```python
from build123d import *

# Parameters (mm, degrees)
F0_W     = 9
F0_H     = 15
F0_W_2   = 3.2
F1_DEPTH = 9
F3_SIZE  = 2


# Not quite as in the source:
# - a feature names something its author has since deleted; it is built from what else it names


with BuildPart() as f1:
    # F0 (on Top) → F1 (new body, symmetric)
    with BuildSketch(Plane.XY):
        with Locations((-4.5, -7.5)):
            Rectangle(F0_W, F0_H)
        with Locations((1.6, -7.5)):
            Rectangle(F0_W_2, F0_H)
        with BuildLine():
            Line((41, 0), (3.2, 0))
            Line((3.2, 0), (3.2, -15))
            Line((3.2, -15), (41, -15))
            ThreePointArc((41, -15), (62.2132034356, -6.2132034356), (71, 15))
            Line((71, 15), (71, 85))
            ThreePointArc((71, 85), (62.2132034356, 106.2132034356), (41, 115))
            Line((41, 115), (-9, 115))
            Line((-9, 115), (-9, 100))
            Line((-9, 100), (41, 100))
            ThreePointArc((41, 100), (51.6066017178, 95.6066017178), (56, 85))
            Line((56, 85), (56, 15))
            ThreePointArc((56, 15), (51.6066017178, 4.3933982822), (41, 0))
        make_face()
    extrude(amount=F1_DEPTH, both=True)

    # F0 (on Top) → F2 (revolve, cut)
    with BuildSketch(Plane.XY):
        with Locations((1.6, -7.5)):
            Rectangle(F0_W_2, F0_H)
    revolve(axis=Axis((0, -7.5, 0), (0, -1, 0)), mode=Mode.SUBTRACT)

    # F3
    f3_edges = [f1.edges().sort_by_distance(p)[0] for p in [
        (-9, -7.5, 9),
        (16, -15, 9),
        (62.213203, -6.213203, 9),
        (71, 50, 9),
        (62.213203, 106.213203, 9),
        (16, 115, 9),
        (-9, 107.5, 9),
        (16, 100, 9),
        (51.606602, 95.606602, 9),
        (56, 50, 9),
        (51.606602, 4.393398, 9),
        (16, 0, 9),
        (-9, -7.5, -9),
        (16, -15, -9),
        (62.213203, -6.213203, -9),
        (71, 50, -9),
        (62.213203, 106.213203, -9),
        (16, 115, -9),
        (-9, 107.5, -9),
        (16, 100, -9),
        (51.606602, 95.606602, -9),
        (56, 50, -9),
        (51.606602, 4.393398, -9),
        (16, 0, -9),
        (-9, -15, 0),
        (-9, 0, 0),
        (-9, 115, 0),
        (-9, 100, 0),
        (-3.2, -15, 0),
        (-3.2, 0, 0),
    ]]
    chamfer(f3_edges, length=F3_SIZE)


solid = f1.part
```
The model under review builds one solid part; all positions refer to its coordinate system, in mm. A direction names the side the tool comes from. Round coordinates to 2 decimals unless told otherwise and drop trailing zeros. Write each loop counter-clockwise with the first axis right and the second up, starting at its lowest first coordinate (ties: lowest second). Pieces come first, ordered by that corner, then holes.
(1) Wall thickness on L1, parallel to Y at x = 10.5, z = -2.75; L2, parallel to Z at x = 0, y = -5.5; L3, parallel to Y at x = 42.5, z = -7.75: over which ranges is each line inside the solid? List them lowest first.
(2) Mouldability with a two-part tool opening along Y and no side actions: class faces 4 (the conical face through (60.803, -5.244, -8.681)), 5 (the flat face through (56, 50, 0)), 6 (the flat face through (71, 50, 0)) as +Y half, -Y half, draft (parallel to the pull), parting line (faces both ways), or undercut.
(3) We need section A-A on x = 10. Give the boundary of the cut face in (y, z), and give its area (3 significant figures).
(4) We need section B-B on z = 0. Give the boundary of the cut face in (x, y), and give its area (3 significant figures).
(5) Insertion check: pin 1 (5 mm diameter, centred on y = 97, z = -5.5, fed in from +X); pin 2 (5 mm diameter, centred on y = 4.5, z = -2, fed in from +X); pin 3 (7 mm diameter, centred on y = 45, z = -3, fed in from -X). Each pin has a flat end and moves straight along its axis. Give the tip position at first contact, or say it passes through.
(6) We need section C-C on x = 0. Give the boundary of the cut face in (y, z), and give its area (3 significant figures).
(7) Machinability: for faces 1 (the cylindrical face through (-2.539, -7.423, -1.947)), 2 (the conical face through (51.713, 95.951, -7.319)), 3 (the cylindrical face through (51.72, 4.51, 0.1)), which of the approach directions +Z, -Z, +X, -X, +Y, -Y give a long, thin tool a straight path to every point of the face, cutting with its end or side? Answer none if there is none.
(8) We need section D-D on y = 37. Give the boundary of the cut face in (x, z).
Findings below:
1. L1: y = -15 to 0, 100 to 115
1. L2: z = -9 to -3.2, 3.2 to 9
1. L3: y = -14.21 to -0.68, 100.68 to 114.21
2. face 4: -Y half
2. face 5: undercut
2. face 6: draft
3. outline: (-15, -7) - (-13, -9) - (-2, -9) - (0, -7) - (0, 7) - (-2, 9) - (-13, 9) - (-15, 7) - close; (100, -7) - (102, -9) - (113, -9) - (115, -7) - (115, 7) - (113, 9) - (102, 9) - (100, 7) - close
3. area: 524 mm2
4. outline: (-9, -13) - (-7, -15) - (-5.2, -15) - (-3.2, -13) - (-3.2, -2) - (-5.2, 0) - (-7, 0) - (-9, -2) - close; (-9, 102) - (-7, 100) - (41, 100) arc R15 cw to (56, 85) - (56, 15) arc R15 cw to (41, 0) - (5.2, 0) - (3.2, -2) - (3.2, -13) - (5.2, -15) - (41, -15) arc R30 ccw to (71, 15) - (71, 85) arc R30 ccw to (41, 115) - (-7, 115) - (-9, 113) - close
4. area: 3,500 mm2
5. pin 1: stops at x = 69.46
5. pin 2: stops at x = 69.91
5. pin 3: stops at x = 56
6. outline: (-15, -7) - (-13, -9) - (-2, -9) - (0, -7) - (0, -5.2) - (-2, -3.2) - (-13, -3.2) - (-15, -5.2) - close; (-15, 5.2) - (-13, 3.2) - (-2, 3.2) - (0, 5.2) - (0, 7) - (-2, 9) - (-13, 9) - (-15, 7) - close; (100, -7) - (102, -9) - (113, -9) - (115, -7) - (115, 7) - (113, 9) - (102, 9) - (100, 7) - close
6. area: 420 mm2
7. face 1: -Y
7. face 2: -Z, -X
7. face 3: +Z, -Z, -X
8. outline: (56, -7) - (58, -9) - (69, -9) - (71, -7) - (71, 7) - (69, 9) - (58, 9) - (56, 7) - close
